Check sheet for the modelled part. Datum: model origin and axes. Units: mm. Round coordinates to 2 decimals unless told otherwise and drop trailing zeros. Order: outer loops, then holes, each group sorted by start corner. A loop starts at its lowest first (then second) coordinate and runs counter-clockwise, first axis right, second up.
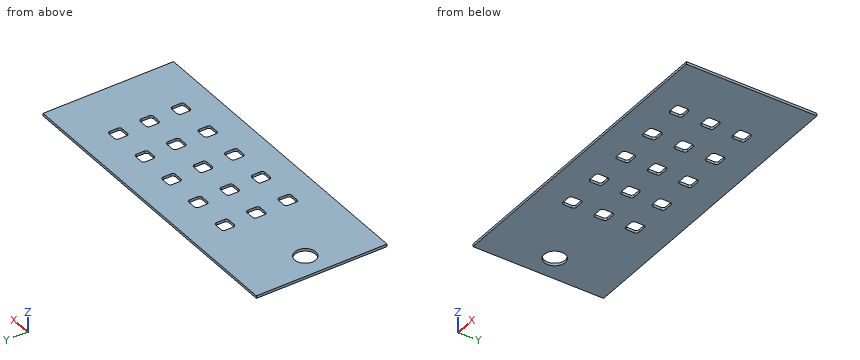
```python
from build123d import *

# Parameters (mm, degrees)
F0_W     = 120
F0_H     = 50
F0_R     = 4
F1_DEPTH = 1


with BuildPart() as f1:
    # F0 (on Top) → F1 (new body)
    with BuildSketch(Plane.XY):
        Rectangle(F0_W, F0_H)
        with BuildLine():
            Line((-21, -15), (-24, -15))
            ThreePointArc((-24, -15), (-24.707107, -14.707107), (-25, -14))
            Line((-25, -14), (-25, -11))
            ThreePointArc((-25, -11), (-24.707107, -10.292893), (-24, -10))
            Line((-24, -10), (-21, -10))
            ThreePointArc((-21, -10), (-20.292893, -10.292893), (-20, -11))
            Line((-20, -11), (-20, -14))
            ThreePointArc((-20, -14), (-20.292893, -14.707107), (-21, -15))
        make_face(mode=Mode.SUBTRACT)
        with BuildLine():
            ThreePointArc((-10, -11), (-9.707107, -10.292893), (-9, -10))
            Line((-9, -10), (-6, -10))
            ThreePointArc((-6, -10), (-5.292893, -10.292893), (-5, -11))
            Line((-5, -11), (-5, -14))
            ThreePointArc((-5, -14), (-5.292893, -14.707107), (-6, -15))
            Line((-6, -15), (-9, -15))
            ThreePointArc((-9, -15), (-9.707107, -14.707107), (-10, -14))
            Line((-10, -14), (-10, -11))
        make_face(mode=Mode.SUBTRACT)
        with BuildLine():
            ThreePointArc((-25, 1), (-24.707107, 1.707107), (-24, 2))
            Line((-24, 2), (-21, 2))
            ThreePointArc((-21, 2), (-20.292893, 1.707107), (-20, 1))
            Line((-20, 1), (-20, -2))
            ThreePointArc((-20, -2), (-20.292893, -2.707107), (-21, -3))
            Line((-21, -3), (-24, -3))
            ThreePointArc((-24, -3), (-24.707107, -2.707107), (-25, -2))
            Line((-25, -2), (-25, 1))
        make_face(mode=Mode.SUBTRACT)
        with BuildLine():
            ThreePointArc((-10, 1), (-9.707107, 1.707107), (-9, 2))
            Line((-9, 2), (-6, 2))
            ThreePointArc((-6, 2), (-5.292893, 1.707107), (-5, 1))
            Line((-5, 1), (-5, -2))
            ThreePointArc((-5, -2), (-5.292893, -2.707107), (-6, -3))
            Line((-6, -3), (-9, -3))
            ThreePointArc((-9, -3), (-9.707107, -2.707107), (-10, -2))
            Line((-10, -2), (-10, 1))
        make_face(mode=Mode.SUBTRACT)
        with BuildLine():
            ThreePointArc((5, -11), (5.292893, -10.292893), (6, -10))
            Line((6, -10), (9, -10))
            ThreePointArc((9, -10), (9.707107, -10.292893), (10, -11))
            Line((10, -11), (10, -14))
            ThreePointArc((10, -14), (9.707107, -14.707107), (9, -15))
            Line((9, -15), (6, -15))
            ThreePointArc((6, -15), (5.292893, -14.707107), (5, -14))
            Line((5, -14), (5, -11))
        make_face(mode=Mode.SUBTRACT)
        with BuildLine():
            ThreePointArc((20, -11), (20.292893, -10.292893), (21, -10))
            Line((21, -10), (24, -10))
            ThreePointArc((24, -10), (24.707107, -10.292893), (25, -11))
            Line((25, -11), (25, -14))
            ThreePointArc((25, -14), (24.707107, -14.707107), (24, -15))
            Line((24, -15), (21, -15))
            ThreePointArc((21, -15), (20.292893, -14.707107), (20, -14))
            Line((20, -14), (20, -11))
        make_face(mode=Mode.SUBTRACT)
        with BuildLine():
            ThreePointArc((5, 1), (5.292893, 1.707107), (6, 2))
            Line((6, 2), (9, 2))
            ThreePointArc((9, 2), (9.707107, 1.707107), (10, 1))
            Line((10, 1), (10, -2))
            ThreePointArc((10, -2), (9.707107, -2.707107), (9, -3))
            Line((9, -3), (6, -3))
            ThreePointArc((6, -3), (5.292893, -2.707107), (5, -2))
            Line((5, -2), (5, 1))
        make_face(mode=Mode.SUBTRACT)
        with BuildLine():
            ThreePointArc((20, 1), (20.292893, 1.707107), (21, 2))
            Line((21, 2), (24, 2))
            ThreePointArc((24, 2), (24.707107, 1.707107), (25, 1))
            Line((25, 1), (25, -2))
            ThreePointArc((25, -2), (24.707107, -2.707107), (24, -3))
            Line((24, -3), (21, -3))
            ThreePointArc((21, -3), (20.292893, -2.707107), (20, -2))
            Line((20, -2), (20, 1))
        make_face(mode=Mode.SUBTRACT)
        with BuildLine():
            ThreePointArc((35, -11), (35.292893, -10.292893), (36, -10))
            Line((36, -10), (39, -10))
            ThreePointArc((39, -10), (39.707107, -10.292893), (40, -11))
            Line((40, -11), (40, -14))
            ThreePointArc((40, -14), (39.707107, -14.707107), (39, -15))
            Line((39, -15), (36, -15))
            ThreePointArc((36, -15), (35.292893, -14.707107), (35, -14))
            Line((35, -14), (35, -11))
        make_face(mode=Mode.SUBTRACT)
        with BuildLine():
            ThreePointArc((35, 1), (35.292893, 1.707107), (36, 2))
            Line((36, 2), (39, 2))
            ThreePointArc((39, 2), (39.707107, 1.707107), (40, 1))
            Line((40, 1), (40, -2))
            ThreePointArc((40, -2), (39.707107, -2.707107), (39, -3))
            Line((39, -3), (36, -3))
            ThreePointArc((36, -3), (35.292893, -2.707107), (35, -2))
            Line((35, -2), (35, 1))
        make_face(mode=Mode.SUBTRACT)
        with Locations((-50.762694, 0)):
            Circle(F0_R, mode=Mode.SUBTRACT)
        with BuildLine():
            ThreePointArc((-25, 13), (-24.707107, 13.707107), (-24, 14))
            Line((-24, 14), (-21, 14))
            ThreePointArc((-21, 14), (-20.292893, 13.707107), (-20, 13))
            Line((-20, 13), (-20, 10))
            ThreePointArc((-20, 10), (-20.292893, 9.292893), (-21, 9))
            Line((-21, 9), (-24, 9))
            ThreePointArc((-24, 9), (-24.707107, 9.292893), (-25, 10))
            Line((-25, 10), (-25, 13))
        make_face(mode=Mode.SUBTRACT)
        with BuildLine():
            ThreePointArc((-10, 13), (-9.707107, 13.707107), (-9, 14))
            Line((-9, 14), (-6, 14))
            ThreePointArc((-6, 14), (-5.292893, 13.707107), (-5, 13))
            Line((-5, 13), (-5, 10))
            ThreePointArc((-5, 10), (-5.292893, 9.292893), (-6, 9))
            Line((-6, 9), (-9, 9))
            ThreePointArc((-9, 9), (-9.707107, 9.292893), (-10, 10))
            Line((-10, 10), (-10, 13))
        make_face(mode=Mode.SUBTRACT)
        with BuildLine():
            ThreePointArc((5, 13), (5.292893, 13.707107), (6, 14))
            Line((6, 14), (9, 14))
            ThreePointArc((9, 14), (9.707107, 13.707107), (10, 13))
            Line((10, 13), (10, 10))
            ThreePointArc((10, 10), (9.707107, 9.292893), (9, 9))
            Line((9, 9), (6, 9))
            ThreePointArc((6, 9), (5.292893, 9.292893), (5, 10))
            Line((5, 10), (5, 13))
        make_face(mode=Mode.SUBTRACT)
        with BuildLine():
            ThreePointArc((20, 13), (20.292893, 13.707107), (21, 14))
            Line((21, 14), (24, 14))
            ThreePointArc((24, 14), (24.707107, 13.707107), (25, 13))
            Line((25, 13), (25, 10))
            ThreePointArc((25, 10), (24.707107, 9.292893), (24, 9))
            Line((24, 9), (21, 9))
            ThreePointArc((21, 9), (20.292893, 9.292893), (20, 10))
            Line((20, 10), (20, 13))
        make_face(mode=Mode.SUBTRACT)
        with BuildLine():
            ThreePointArc((35, 13), (35.292893, 13.707107), (36, 14))
            Line((36, 14), (39, 14))
            ThreePointArc((39, 14), (39.707107, 13.707107), (40, 13))
            Line((40, 13), (40, 10))
            ThreePointArc((40, 10), (39.707107, 9.292893), (39, 9))
            Line((39, 9), (36, 9))
            ThreePointArc((36, 9), (35.292893, 9.292893), (35, 10))
            Line((35, 10), (35, 13))
        make_face(mode=Mode.SUBTRACT)
    extrude(amount=F1_DEPTH)


solid = f1.part
```
Item 1: Scan lines: line 1 along X through (y, z) = (13, 0.2); line 2 along Y through (x, z) = (39, 0.5); line 3 along Y through (x, z) = (24.5, 0.2). Record each from-to range of solid material in increasing order.
Answer:
line 1: x = -60 to -25, -20 to -10, -5 to 5, 10 to 20, 25 to 35, 40 to 60
line 2: y = -25 to -15, -10 to -3, 2 to 9, 14 to 25
line 3: y = -25 to -14.87, -10.13 to -2.87, 1.87 to 9.13, 13.87 to 25
Item 2: Sectioned sample at A-A (x = 7.5). Record the cut outline in (y, z).
Answer:
outline: (-25, 0) - (-15, 0) - (-15, 1) - (-25, 1) - close; (-10, 0) - (-3, 0) - (-3, 1) - (-10, 1) - close; (2, 0) - (9, 0) - (9, 1) - (2, 1) - close; (14, 0) - (25, 0) - (25, 1) - (14, 1) - close
Item 3: Go/stop test with a flat-tipped pin: P1, Ø3, axis at x = 8.5, y = 4, coming from the -Z side. Record where the tip stops, or that it passes through.
Answer:
P1: stops at z = 0
Item 4: Sectioned sample at B-B (z = 0.55). State how many separate pieces and enclosed holes the cut face has, and give its area (3 significant figures).
Answer:
separate pieces: 1
enclosed holes: 16
area: 5,590 mm2
